from build123d import *

# Parameters (mm, degrees)
SKETCH5_W                   = 15
SKETCH5_H                   = 7.525
CUT_EXTRUDE_START           = -15
CUT_EXTRUDE_1_OUTLINE_R     = 3.175
CUT_EXTRUDE_1_DEPTH         = 15
CUT_EXTRUDE_START_2         = -21
CUT_EXTRUDE_1_2_OUTLINE_R   = 4
CUT_EXTRUDE_1_2_OUTLINE_R_2 = 3.175
CUT_EXTRUDE_1_2_DEPTH       = 6
CUT_EXTRUDE_START_3         = -14.5
CUT_EXTRUDE_1_3_DEPTH       = 14
CUT_EXTRUDE_START_4         = 2
CUT_EXTRUDE_1_5_OUTLINE_R   = 1.433256124
CUT_EXTRUDE_1_5_DEPTH       = 5.353381724


with BuildPart() as part:
    # Sketch5 → body (revolve)
    with BuildSketch(Plane(origin=(0, 0, 0), x_dir=(0, 0, -1), z_dir=(1, 0, 0)), mode=Mode.PRIVATE) as body_sk:
        with Locations((7.5, 3.7625)):
            Rectangle(SKETCH5_W, SKETCH5_H)
    revolve(body_sk.sketch.rotate(Axis((0, 0, 0), (0, 0, 1)), 270), axis=Axis((0, 0, 0), (0, 0, 1)))

    # Вырез-Вытянуть1: read off the stored shape, not the designer's step
    # Вырез-Вытянуть1 outline → Вырез-Вытянуть1 (cut)
    with BuildSketch(Plane.XY.offset(CUT_EXTRUDE_START)):
        Circle(CUT_EXTRUDE_1_OUTLINE_R)
    extrude(amount=CUT_EXTRUDE_1_DEPTH, mode=Mode.SUBTRACT)

    # Cut-Extrude 1 2 outline → Cut-Extrude 1 2 (add)
    with BuildSketch(Plane.XY.offset(CUT_EXTRUDE_START_2)):
        Circle(CUT_EXTRUDE_1_2_OUTLINE_R)
        Circle(CUT_EXTRUDE_1_2_OUTLINE_R_2, mode=Mode.SUBTRACT)
    extrude(amount=CUT_EXTRUDE_1_2_DEPTH)

    # Cut-Extrude 1 3 outline → Cut-Extrude 1 3 (cut)
    with BuildSketch(Plane.XY.offset(CUT_EXTRUDE_START_3)):
        with BuildLine():
            ThreePointArc((1.178506304, 7.090189781), (1.362296798, 7.304241747), (1.641646979, 7.343747013))
            ThreePointArc((1.641646979, 7.343747013), (0, 7.525), (-1.641646979, 7.343747013))
            ThreePointArc((-1.641646979, 7.343747013), (-1.362296798, 7.304241747), (-1.178506304, 7.090189781))
            Line((-1.178506304, 7.090189781), (-0.995794033, 6.588191943))
            ThreePointArc((-0.995794033, 6.588191943), (-0.84934756, 6.397339182), (-0.619916985, 6.325))
            Line((-0.619916985, 6.325), (0.619916985, 6.325))
            ThreePointArc((0.619916985, 6.325), (0.84934756, 6.397339182), (0.995794033, 6.588191943))
            Line((0.995794033, 6.588191943), (1.178506304, 7.090189781))
        make_face()
        with BuildLine():
            ThreePointArc((5.644666496, 4.976280253), (4.423084023, 6.087852883), (2.988425886, 6.90615202))
            ThreePointArc((2.988425886, 6.90615202), (3.191204317, 6.709993671), (3.214077361, 6.428792651))
            Line((3.214077361, 6.428792651), (3.066827768, 5.915272291))
            ThreePointArc((3.066827768, 5.915272291), (3.073125016, 5.674790087), (3.216218345, 5.481410551))
            Line((3.216218345, 5.481410551), (4.219265096, 4.752654428))
            ThreePointArc((4.219265096, 4.752654428), (4.447398235, 4.676322148), (4.678056359, 4.744646197))
            Line((4.678056359, 4.744646197), (5.120940617, 5.043375401))
            ThreePointArc((5.120940617, 5.043375401), (5.395446839, 5.108517737), (5.644666496, 4.976280253))
        make_face()
        with BuildLine():
            ThreePointArc((-3.214077361, 6.428792651), (-3.191204317, 6.709993671), (-2.988425886, 6.90615202))
            ThreePointArc((-2.988425886, 6.90615202), (-4.423084023, 6.087852883), (-5.644666496, 4.976280253))
            ThreePointArc((-5.644666496, 4.976280253), (-5.395446839, 5.108517737), (-5.120940617, 5.043375401))
            Line((-5.120940617, 5.043375401), (-4.678056359, 4.744646197))
            ThreePointArc((-4.678056359, 4.744646197), (-4.447398235, 4.676322148), (-4.219265096, 4.752654428))
            Line((-4.219265096, 4.752654428), (-3.216218345, 5.481410551))
            ThreePointArc((-3.216218345, 5.481410551), (-3.073125016, 5.674790087), (-3.066827768, 5.915272291))
            Line((-3.066827768, 5.915272291), (-3.214077361, 6.428792651))
        make_face()
        with BuildLine():
            ThreePointArc((7.491615266, 0.708043573), (7.156700285, 2.325352883), (6.477021636, 3.830641686))
            ThreePointArc((6.477021636, 3.830641686), (6.525773848, 3.552756077), (6.378992717, 3.311815235))
            Line((6.378992717, 3.311815235), (5.958025599, 2.982919676))
            ThreePointArc((5.958025599, 2.982919676), (5.821768286, 2.784664057), (5.823867582, 2.544108577))
            Line((5.823867582, 2.544108577), (6.206997349, 1.364956402))
            ThreePointArc((6.206997349, 1.364956402), (6.346693946, 1.169108995), (6.573460157, 1.088806868))
            Line((6.573460157, 1.088806868), (7.107349669, 1.070163036))
            ThreePointArc((7.107349669, 1.070163036), (7.367719572, 0.961513584), (7.491615266, 0.708043573))
        make_face()
        with BuildLine():
            ThreePointArc((-6.378992717, 3.311815235), (-6.525773848, 3.552756077), (-6.477021636, 3.830641686))
            ThreePointArc((-6.477021636, 3.830641686), (-7.156700285, 2.325352883), (-7.491615266, 0.708043573))
            ThreePointArc((-7.491615266, 0.708043573), (-7.367719572, 0.961513584), (-7.107349669, 1.070163036))
            Line((-7.107349669, 1.070163036), (-6.573460157, 1.088806868))
            ThreePointArc((-6.573460157, 1.088806868), (-6.346693946, 1.169108995), (-6.206997349, 1.364956402))
            Line((-6.206997349, 1.364956402), (-5.823867582, 2.544108577))
            ThreePointArc((-5.823867582, 2.544108577), (-5.821768286, 2.784664057), (-5.958025599, 2.982919676))
            Line((-5.958025599, 2.982919676), (-6.378992717, 3.311815235))
        make_face()
        with BuildLine():
            ThreePointArc((6.477021636, -3.830641686), (7.156700285, -2.325352883), (7.491615266, -0.708043573))
            ThreePointArc((7.491615266, -0.708043573), (7.367719572, -0.961513584), (7.107349669, -1.070163036))
            Line((7.107349669, -1.070163036), (6.573460157, -1.088806868))
            ThreePointArc((6.573460157, -1.088806868), (6.346693946, -1.169108995), (6.206997349, -1.364956402))
            Line((6.206997349, -1.364956402), (5.823867582, -2.544108577))
            ThreePointArc((5.823867582, -2.544108577), (5.821768286, -2.784664057), (5.958025599, -2.982919676))
            Line((5.958025599, -2.982919676), (6.378992717, -3.311815235))
            ThreePointArc((6.378992717, -3.311815235), (6.525773848, -3.552756077), (6.477021636, -3.830641686))
        make_face()
        with BuildLine():
            ThreePointArc((-7.107349669, -1.070163036), (-7.367719572, -0.961513584), (-7.491615266, -0.708043573))
            ThreePointArc((-7.491615266, -0.708043573), (-7.156700285, -2.325352883), (-6.477021636, -3.830641686))
            ThreePointArc((-6.477021636, -3.830641686), (-6.525773848, -3.552756077), (-6.378992717, -3.311815235))
            Line((-6.378992717, -3.311815235), (-5.958025599, -2.982919676))
            ThreePointArc((-5.958025599, -2.982919676), (-5.821768286, -2.784664057), (-5.823867582, -2.544108577))
            Line((-5.823867582, -2.544108577), (-6.206997349, -1.364956402))
            ThreePointArc((-6.206997349, -1.364956402), (-6.346693946, -1.169108995), (-6.573460157, -1.088806868))
            Line((-6.573460157, -1.088806868), (-7.107349669, -1.070163036))
        make_face()
        with BuildLine():
            ThreePointArc((2.988425886, -6.90615202), (4.423084023, -6.087852883), (5.644666496, -4.976280253))
            ThreePointArc((5.644666496, -4.976280253), (5.395446839, -5.108517737), (5.120940617, -5.043375401))
            Line((5.120940617, -5.043375401), (4.678056359, -4.744646197))
            ThreePointArc((4.678056359, -4.744646197), (4.447398235, -4.676322148), (4.219265096, -4.752654428))
            Line((4.219265096, -4.752654428), (3.216218345, -5.481410551))
            ThreePointArc((3.216218345, -5.481410551), (3.073125016, -5.674790087), (3.066827768, -5.915272291))
            Line((3.066827768, -5.915272291), (3.214077361, -6.428792651))
            ThreePointArc((3.214077361, -6.428792651), (3.191204317, -6.709993671), (2.988425886, -6.90615202))
        make_face()
        with BuildLine():
            ThreePointArc((-5.120940617, -5.043375401), (-5.395446839, -5.108517737), (-5.644666496, -4.976280253))
            ThreePointArc((-5.644666496, -4.976280253), (-4.423084023, -6.087852883), (-2.988425886, -6.90615202))
            ThreePointArc((-2.988425886, -6.90615202), (-3.191204317, -6.709993671), (-3.214077361, -6.428792651))
            Line((-3.214077361, -6.428792651), (-3.066827768, -5.915272291))
            ThreePointArc((-3.066827768, -5.915272291), (-3.073125016, -5.674790087), (-3.216218345, -5.481410551))
            Line((-3.216218345, -5.481410551), (-4.219265096, -4.752654428))
            ThreePointArc((-4.219265096, -4.752654428), (-4.447398235, -4.676322148), (-4.678056359, -4.744646197))
            Line((-4.678056359, -4.744646197), (-5.120940617, -5.043375401))
        make_face()
        with BuildLine():
            ThreePointArc((-1.641646979, -7.343747013), (0, -7.525), (1.641646979, -7.343747013))
            ThreePointArc((1.641646979, -7.343747013), (1.362296798, -7.304241747), (1.178506304, -7.090189781))
            Line((1.178506304, -7.090189781), (0.995794033, -6.588191943))
            ThreePointArc((0.995794033, -6.588191943), (0.84934756, -6.397339182), (0.619916985, -6.325))
            Line((0.619916985, -6.325), (-0.619916985, -6.325))
            ThreePointArc((-0.619916985, -6.325), (-0.84934756, -6.397339182), (-0.995794033, -6.588191943))
            Line((-0.995794033, -6.588191943), (-1.178506304, -7.090189781))
            ThreePointArc((-1.178506304, -7.090189781), (-1.362296798, -7.304241747), (-1.641646979, -7.343747013))
        make_face()
    extrude(amount=CUT_EXTRUDE_1_3_DEPTH, mode=Mode.SUBTRACT)

    # Cut-Extrude 1 4 outline → Cut-Extrude 1 4 (revolve)
    with BuildSketch(Plane.XZ):
        Polygon((7.525, 0), (7.525, -0.5), (7.658974596, -0.5), (9.75, 0.060288568), (9.616025404, 0.560288568), align=None)
        Polygon((7.658974596, -14.5), (7.525, -14.5), (7.525, -15), (9.616025404, -15.560288568), (9.75, -15.060288568), align=None)
    revolve(axis=Axis((0, 0, 0), (0, 0, 1)))

    # Cut-Extrude 1 5 outline → Cut-Extrude 1 5 (cut)
    with BuildSketch(Plane(origin=(0, 0, 0), x_dir=(1, 0, 0), z_dir=(0, 1, 0)).offset(CUT_EXTRUDE_START_4)):
        with Locations((0, 8)):
            Circle(CUT_EXTRUDE_1_5_OUTLINE_R)
    extrude(amount=CUT_EXTRUDE_1_5_DEPTH, mode=Mode.SUBTRACT)


solid = part.part
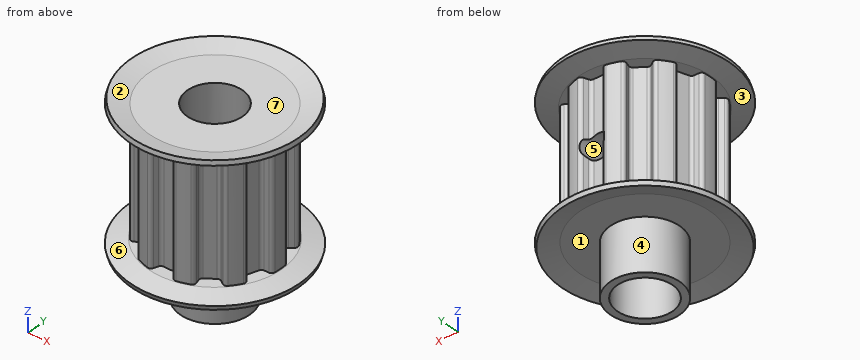
CAD build for the part. Positions are in the model's coordinates, mm. Face numbers are marked on the shaded views. A direction names the side the tool comes from. Round coordinates to 2 decimals unless told otherwise and drop trailing zeros. Write each loop counter-clockwise with the first axis right and the second up, starting at its lowest first coordinate (ties: lowest second). Pieces come first, ordered by that corner, then holes.
(1) Mould opens along Z. For the marked faces 1, 2 and 3 say: pulls with the +Z half, pulls with the -Z half, needs draft (parallel to the pull), parting line crosses it, or undercut.
(2) Probe line 1 along Y through (x, z) = (0, -3.5) (3 decimals); line 2 along Z through (x, y) = (-4.5, 5.25); line 3 along Z through (x, y) = (0, 5.8). List the from-to ranges inside material, lowest first.
(3) Slice it at A-A, the plane x = 0. Count the separate pieces of the cut face and the enclosed holes in it, and give its area (3 significant figures).
(4) Drop flat-ended pins along their axis: P1, Ø1.5, axis at y = 7, z = -8, coming from the -X side; P2, Ø0.6, axis at x = 0, z = -12.5, coming from the +Y side (3 decimals); P3, Ø1.5, axis at y = 7.5, z = -11.5, coming from the +X side; P4, Ø5.5, axis at x = 0, y = 0, coming from the +Z side. Give the stop position or say it passes through.
(5) 3-axis set-ups, long thin cutter, end or side, ignore diameter. For the marked faces 4, 5, 6 and 7: which of +Z, -Z, +X, -X, +Y, -Y reach the whole face in a straight line?
(6) Slice it at C-C, the plane z = -18.75. Write the cut outline in (x, y) (3 decimals), and give its area (3 significant figures).
(7) Slice it at B-B, the plane y = 0. Write the cut outline in (x, z) (3 decimals), and give its area (3 significant figures).
From the geometry:
1. face 1: pulls with the -Z half
1. face 2: pulls with the +Z half
1. face 3: undercut
2. line 1: y = -6.325 to -3.175, 3.175 to 6.325
2. line 2: z = -15 to -14.5, -0.5 to 0
2. line 3: z = -15 to -9.43, -6.57 to 0
3. separate pieces: 3
3. enclosed holes: 0
3. area: 102 mm2
4. P1: stops at x = -3.23
4. P2: stops at y = 6.325
4. P3: stops at x = 3.17
4. P4: passes through
5. face 4: -Z
5. face 5: +Y
5. face 6: none
5. face 7: +Z
6. outline: circle Ø8 at (0, 0); hole circle Ø6.35 at (0, 0)
6. area: 18.6 mm2
7. outline: (-9.75, -15.06) - (-9.616, -15.56) - (-7.525, -15) - (-4, -15) - (-4, -21) - (-3.175, -21) - (-3.175, 0) - (-7.525, 0) - (-9.616, 0.56) - (-9.75, 0.06) - (-7.659, -0.5) - (-7.525, -0.5) - (-7.525, -14.5) - (-7.659, -14.5) - close; (3.175, -21) - (4, -21) - (4, -15) - (7.525, -15) - (9.616, -15.56) - (9.75, -15.06) - (7.659, -14.5) - (7.525, -14.5) - (7.525, -0.5) - (7.659, -0.5) - (9.75, 0.06) - (9.616, 0.56) - (7.525, 0) - (3.175, 0) - close
7. area: 145 mm2
